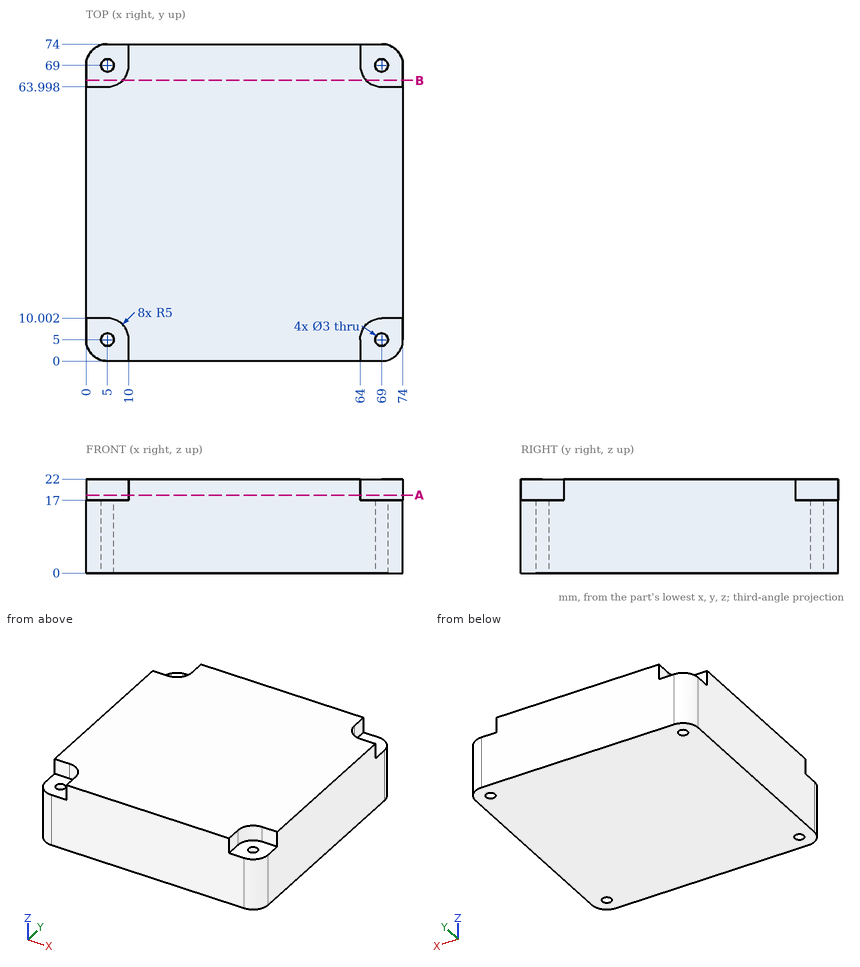
Print and shaded views of the part. All mm, measured from the part's lowest x, y and z. Give positions to 0.01 mm unless a question says otherwise; leave off trailing zeros. Order: outer loops, then holes, each group sorted by start corner. A loop starts at its lowest first (then second) coordinate and runs counter-clockwise, first axis right, second up. Notation, with made-up numbers: (-15.75, -23.5) - (-7.75, -23.5) arc R15 ccw to (-7.75, -19.5) - close; hole circle Ø8 at (17.5, -37.75). An arc over 180 degrees is marked (long way). One line per item, written item: value.
Item 1: Slice it at B-B (y = 65.5). List the corners of the cut face in (x, z).
Response values:
outline: (0, 0) - (74, 0) - (74, 17) - (65.43, 17) - (65.43, 22) - (8.57, 22) - (8.57, 17) - (0, 17) - close
Item 2: Slice it at A-A (z = 18.25). List the corners of the cut face in (x, y), then the cut area to 3 significant figures.
Response values:
outline: (0, 10) - (5, 10) arc R5 cw to (10, 5) - (10, 0) - (64, 0) - (64, 5) arc R5 cw to (69, 10) - (74, 10) - (74, 64) - (69, 64) arc R5 cw to (64, 69) - (64, 74) - (10, 74) - (10, 69) arc R5 cw to (5, 64) - (0, 64) - close
area: 5,100 mm2
Item 3: Pin check, flat tips, straight feed: pin 1 Ø10 at (y, z) = (56.5, 19) entering from -X; pin 2 Ø5.5 at (x, z) = (70.5, 20.5) entering from +Y; pin 3 Ø3.5 at (x, y) = (5, 5) entering from +Z; pin 4 Ø2.5 at (x, z) = (71, 19) entering from -Y. Stop position of each tip, or through.
Response values:
pin 1: x = 0
pin 2: y = 64.16
pin 3: z = 17
pin 4: y = 10
Item 4: Wall check: line 1 (X direction, y = 70, z = 4.5); line 2 (Y direction, x = 65, z = 19.25). Give the ranges that are in metal, low to high.
Response values:
line 1: 0.1 to 3.88, 6.12 to 67.88, 70.12 to 73.9
line 2: 8 to 66
